from build123d import *

# Parameters (mm, degrees)
SKETCH1_R           = 75
BOSS_EXTRUDE1_DEPTH = 40
BOSS_EXTRUDE2_DEPTH = 30
SKETCH3_R           = 75
BOSS_EXTRUDE3_DEPTH = 40


with BuildPart() as part:
    # Sketch1 → Boss-Extrude1 (new body)
    with BuildSketch(Plane(origin=(0, 0, 0), x_dir=(0, 0, -1), z_dir=(1, 0, 0))):
        Circle(SKETCH1_R)
    extrude(amount=BOSS_EXTRUDE1_DEPTH)

    # Sketch2 → Boss-Extrude2 (add)
    with BuildSketch(Plane(origin=(40, 0, 0), x_dir=(0, 0, -1), z_dir=(1, 0, 0))):
        with BuildLine():
            Line((0, 40), (300, 40))
            ThreePointArc((300, 40), (340, 0), (300, -40))
            Line((300, -40), (0, -40))
            ThreePointArc((0, -40), (-40, 0), (0, 40))
        make_face()
    extrude(amount=BOSS_EXTRUDE2_DEPTH)

    # Sketch3 → Boss-Extrude3 (add)
    with BuildSketch(Plane.ZY.offset(-40)):
        with Locations((-300, 0)):
            Circle(SKETCH3_R)
    extrude(amount=BOSS_EXTRUDE3_DEPTH)


solid = part.part
Work out the finished part from the listing and answer in its coordinate system (mm). A direction names the side the tool comes from. Give positions to 0.01 mm unless a question says otherwise; leave off trailing zeros. Loops run counter-clockwise (first coordinate to the right, second up) from the corner with the lowest first, then second, coordinate; pieces in that order, holes last. Notation, with made-up numbers: (10.5, -5) -> (42.5, -5) arc R22 cw to (42.5, 2) -> close; hole circle Ø6 at (64.25, 38). An arc over 180 degrees is marked (long way). Use a Markdown table: item, result. Add a question column.
1) Which of the six approach directions +Z, -Z, +X, -X, +Y, -Y give full straight-line access (tool end or side, diameter ignored) to faces 1 (the cylindrical face through (20.28, 22.528, -228.463)), 2 (the flat face through (55, -40, -152)), 3 (the flat face through (55, 40, -148)), 4 (the cylindrical face through (54.79, -0.88, 39.99)), 5 (the flat face through (40, 18, -338))?
2) Each of these flat-tipped pins is pushed along its axis until it touches: P1, Ø2, axis at x = 11, y = 16.5, coming from the -Z side; P2, Ø9, axis at x = 56.5, z = -142, coming from the +Y side; P3, Ø1.5, axis at x = 28.5, y = 48, coming from the +Z side. Where does it stop, or does it pass through?
3) The part is cut by section A-A, the plane y = 45.5. Determine the outline of the cut face in (x, z), plus the area to 3 significant figures.
4) The part is cut by section C-C, the plane x = 26.5. Determine the outline of the cut face in (y, z), plus the area to 3 significant figures.
5) Consider line 1 along Z through (x, y) = (18, -2.5); line 2 along Y through (x, z) = (47, -81.5); line 3 along Z through (x, y) = (7.5, -48.5). Determine where each line is inside the solid, lowest interval first.
6) The part is cut by section B-B, the plane y = 0. Determine the outline of the cut face in (x, z).
7) The part is cut by section D-D, the plane z = -30. Determine the outline of the cut face in (x, y), plus the area to 3 significant figures.
Reported:
| question | item | result |
|---|---|---|
| 1 | face 1 | -X |
| 1 | face 2 | +Z, -Z, +X, -Y |
| 1 | face 3 | +Z, -Z, +X, +Y |
| 1 | face 4 | +Z, +X |
| 1 | face 5 | -Z, +X |
| 2 | P1 | stops at z = -373.38 |
| 2 | P2 | stops at y = 40 |
| 2 | P3 | stops at z = 58.24 |
| 3 | outline | (0, -359.62) -> (40, -359.62) -> (40, -240.38) -> (0, -240.38) -> close; (0, -59.62) -> (40, -59.62) -> (40, 59.62) -> (0, 59.62) -> close |
| 3 | area | 9,540 mm^2 |
| 4 | outline | circle Ø150 at (0, -300); circle Ø150 at (0, 0) |
| 4 | area | 35,300 mm^2 |
| 5 | line 1 | z = -374.96 to -225.04, -74.96 to 74.96 |
| 5 | line 2 | y = -40 to 40 |
| 5 | line 3 | z = -357.21 to -242.79, -57.21 to 57.21 |
| 6 | outline | (0, -375) -> (40, -375) -> (40, -340) -> (70, -340) -> (70, 40) -> (40, 40) -> (40, 75) -> (0, 75) -> (0, -75) -> (40, -75) -> (40, -225) -> (0, -225) -> close |
| 7 | outline | (0, -68.74) -> (40, -68.74) -> (40, -40) -> (70, -40) -> (70, 40) -> (40, 40) -> (40, 68.74) -> (0, 68.74) -> close |
| 7 | area | 7,900 mm^2 |
